Can you work these out from the drawing? Everything is in mm from the part's minimum corner. A direction names the side the tool comes from. Coordinates: 2 decimals unless noted, no trailing zeros. Order: outer loops, then holes, each group sorted by start corner. A loop starts at its lowest first (then second) coordinate and runs counter-clockwise, first axis right, second up. Notation, with made-up numbers: (65.25, 39) - (114.25, 39) arc R10 ccw to (114.25, 56) - close; hole circle Ø1 at (73.5, 49). An arc over 180 degrees is marked (long way). Use CSV: the item, a comma, the result in double quotes. Start each with the question number.
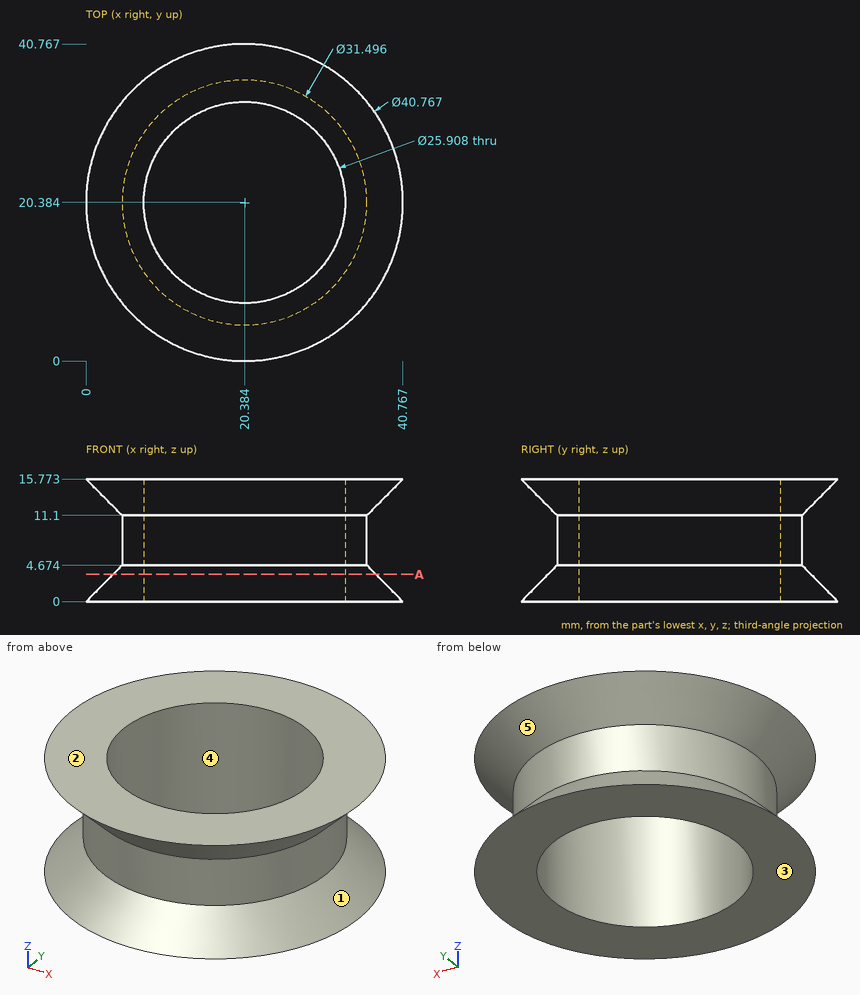
Item 1: Suppose I cut it at A-A on z = 3.5. Write out the boundary of the cut face in (x, y) (1 decimal).
Item 2: For the marked faces 1 and 2, which set-ups out of +Z, -Z, +X, -X, +Y, -Y let a thin tool reach every point of the face, with its end or its side?
Item 3: We'd pull the mould along Z, two halves only. Please class the marked faces 3, 4 and 5: released by +Z, released by -Z, zero draft, split by the parting line, or undercut.
Item 4: Please list where these lines run through material, in increasing order: line 1 along Y through (x, z) = (20.5, 10.25) (1 decimal); line 2 along Z through (x, y) = (4.5, 15.5) (1 decimal); line 3 along X through (y, z) = (14.5, 14.75) (1 decimal). Write a range as from..to.
Item 5: For pin 1 Ø1 at (x, z) = (9.5, 10.5) entering from +Y (1 decimal); pin 2 Ø1.5 at (y, z) = (10, 7) entering from -X (1 decimal); pin 3 Ø3 at (x, z) = (32, 3.5) entering from -Y (1 decimal), each with a flat end and sliding along its axis, tell me the tip position at first contact or that it passes through.
Here are the results:
1,outline,"circle Ø33.8 at (20.4, 20.4); hole circle Ø25.9 at (20.4, 20.4)"
2,face 1,"none"
2,face 2,"+Z, +X, -X, +Y, -Y"
3,face 3,"released by -Z"
3,face 4,"zero draft"
3,face 5,"undercut"
4,line 1,"4.6..7.4, 33.3..36.1"
4,line 2,"0..3.8, 12..15.8"
4,line 3,"1.9..8.8, 31.9..38.8"
5,pin 1,"y = 32.2"
5,pin 2,"x = 7.9"
5,pin 3,"y = 5.8"
